Geometry: final body of the model. Coordinates: model frame, mm. A direction names the side the tool comes from. Coordinates: 2 decimals unless noted, no trailing zeros. Order: outer loops, then holes, each group sorted by start corner. A loop starts at its lowest first (then second) coordinate and runs counter-clockwise, first axis right, second up. Notation, with made-up numbers: M 11.25,-13 L 42.25,-13 A29 ccw 42.25,24 Z; hole C 53,-21.5 d9. An arc over 180 degrees is marked long. Use CSV: the item, a comma, the result in double quotes. Start each with the question number.
1. First-contact query: P1, Ø4, axis at x = -27.05, y = 7.43, coming from the -Z side; P2, Ø1.5, axis at y = 1.5, z = 12.5, coming from the -X side; P3, Ø1, axis at x = -8, y = 7.5, coming from the +Z side. Flat tips, straight axial feed; report the tip coordinate or a pass-through.
2. Material intervals for line 1 (Z direction, x = -22.5, y = 14.25); line 2 (Y direction, x = -28.5, z = 12.5); line 3 (X direction, y = -1, z = 9.25), sorted ascending.
3. Section query A-A on z = 13.25. Return the cut outline in (x, y) (1 decimal).
4. Set-up query: faces 1 (the cylindrical face through (-4.2, 11.63, 7.91)), 2 (the flat face through (-8, 7, 7)). Return all of +Z, -Z, +X, -X, +Y, -Y with unobstructed straight access to the full face (end or side cutting, diameter ignored); none if empty.
5. Section query B-B on z = 2.75. Return the cut outline in (x, y), and give its area (3 significant figures).
6. Pull-direction query (X, two-part tool) for faces 3 (the cylindrical face through (-19.764, 5.398, -2.218)), 4 (the flat face through (-18, 15, 7)), 5 (the flat face through (-15, 5, 0)); classes: pulls with the +X half, pulls with the -X half, needs draft (parallel to the pull), parting line crosses it, or undercut.
from build123d import *

# Parameters (mm, degrees)
SKETCH1_R           = 14
BOSS_EXTRUDE1_DEPTH = 17
SKETCH2_R           = 3
BOSS_EXTRUDE2_DEPTH = 5
SKETCH3_R           = 1.5875
CUT_EXTRUDE2_DEPTH  = 10
CHAMFER1_SIZE       = 1.5
CHAMFER2_SIZE       = 0.5
CHAMFER3_SIZE       = 2.5


with BuildPart() as part:
    # Sketch1 → Boss-Extrude1 (new body)
    with BuildSketch(Plane.XY):
        with Locations((-17.5533458, 7.425814207)):
            Circle(SKETCH1_R)
    extrude(amount=BOSS_EXTRUDE1_DEPTH)

    # Sketch2 → Boss-Extrude2 (add)
    with BuildSketch(Plane(origin=(0, -0.075436545, 0), x_dir=(-1, 0, 0), z_dir=(0, 0, -1))):
        with Locations(Location((17.5533458, 7.501250752, 0), (0, 0, 180))):
            Circle(SKETCH2_R)
    extrude(amount=BOSS_EXTRUDE2_DEPTH)

    # Sketch3 → Cut-Extrude2 (cut)
    with BuildSketch(Plane.XY.offset(17)):
        with Locations((-27.0533458, 7.425814207)):
            Circle(SKETCH3_R)
        with Locations((-17.5533458, -0.574185793)):
            Circle(SKETCH3_R)
        with Locations((-8.0533458, 7.425814207)):
            Circle(SKETCH3_R)
        with Locations((-17.5533458, 15.425814207)):
            Circle(SKETCH3_R)
    extrude(amount=-CUT_EXTRUDE2_DEPTH, mode=Mode.SUBTRACT)

    # Chamfer1
    chamfer1_edges = [part.edges().sort_by_distance(p)[0] for p in [
        (-31.5533458, 7.425814207, 0),
    ]]
    chamfer(chamfer1_edges, length=CHAMFER1_SIZE)

    # Chamfer2
    chamfer2_edges = [part.edges().sort_by_distance(p)[0] for p in [
        (-20.5533458, 7.425814207, -5),
    ]]
    chamfer(chamfer2_edges, length=CHAMFER2_SIZE)

    # Chamfer3
    chamfer3_edges = [part.edges().sort_by_distance(p)[0] for p in [
        (-31.5533458, 7.425814207, 17),
    ]]
    chamfer(chamfer3_edges, length=CHAMFER3_SIZE)


solid = part.part
Results list:
1,P1,"stops at z = 0"
1,P2,"stops at x = -30.56"
1,P3,"stops at z = 7"
2,line 1,"z = 0 to 17"
2,line 2,"y = -1.3 to 6.77, 8.08 to 16.15"
2,line 3,"x = -28.73 to -19.08, -16.02 to -6.37"
3,outline,"C -17.6,7.4 d28; hole C -27.1,7.4 d3.2; hole C -17.6,-0.6 d3.2; hole C -17.6,15.4 d3.2; hole C -8.1,7.4 d3.2"
4,face 1,"+Z, -Z"
4,face 2,"+Z"
5,outline,"C -17.55,7.43 d28"
5,area,"616 mm²"
6,face 3,"parting line crosses it"
6,face 4,"undercut"
6,face 5,"needs draft"
